Input: dimensioned drawing with shaded views. Units: mm. Origin: part minimum x, y, z. A direction names the side the tool comes from. Give positions to 0.01 mm unless a question says otherwise; leave off trailing zeros. Write each loop counter-clockwise with the first axis right and the second up, starting at its lowest first coordinate (ties: lowest second). Pieces come first, ordered by that corner, then holes. Notation, with made-up numbers: (-13.5, 88.5) - (-6.5, 88.5) arc R19 ccw to (-6.5, 99.5) - close; hole circle Ø1 at (36.25, -10.5). An arc over 180 degrees is marked (long way). Answer as CSV lines item,"result".
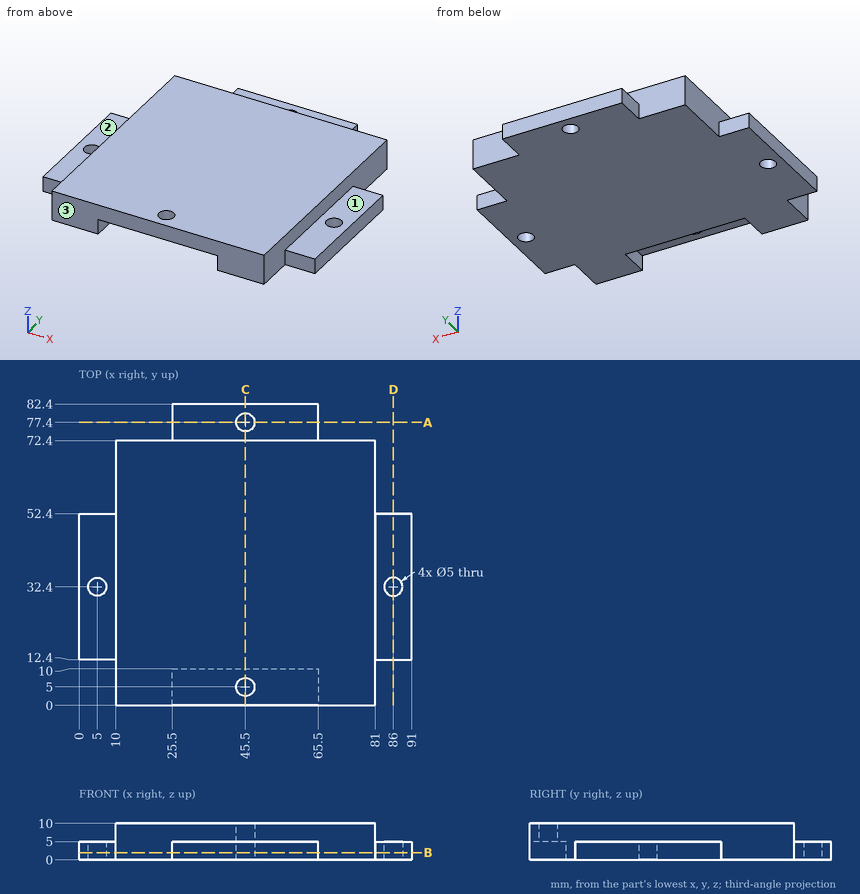
Item 1: Cut plane C-C on x = 45.5. Return the cut outline in (y, z), plus the area to 3 significant figures.
The answers:
outline,"(0, 5) - (2.5, 5) - (2.5, 10) - (0, 10) - close; (7.5, 5) - (10, 5) - (10, 0) - (74.9, 0) - (74.9, 5) - (72.4, 5) - (72.4, 10) - (7.5, 10) - close; (79.9, 0) - (82.4, 0) - (82.4, 5) - (79.9, 5) - close"
area,"674 mm²"
Item 2: Reachability of the marked faces 1, 2 and 3 from +Z, -Z, +X, -X, +Y, -Y: full face, straight path, thin tool, end or side. Return the list, or none.
The answers:
face 1,"+Z, +X, +Y, -Y"
face 2,"+Z, -X, +Y, -Y"
face 3,"+Z, -Z, +X, -X, -Y"
Item 3: Cut plane A-A on y = 77.4. Return the cut outline in (x, z).
The answers:
outline,"(25.5, 0) - (43, 0) - (43, 5) - (25.5, 5) - close; (48, 0) - (65.5, 0) - (65.5, 5) - (48, 5) - close"
Item 4: Cut plane D-D on x = 86. Return the cut outline in (y, z), plus the area to 3 significant figures.
The answers:
outline,"(12.4, 0) - (29.9, 0) - (29.9, 5) - (12.4, 5) - close; (34.9, 0) - (52.4, 0) - (52.4, 5) - (34.9, 5) - close"
area,"175 mm²"
Item 5: Cut plane B-B on z = 2. Return the cut outline in (x, y).
The answers:
outline,"(0, 12.4) - (10, 12.4) - (10, 0) - (25.5, 0) - (25.5, 10) - (65.5, 10) - (65.5, 0) - (81, 0) - (81, 12.4) - (91, 12.4) - (91, 52.4) - (81, 52.4) - (81, 72.4) - (65.5, 72.4) - (65.5, 82.4) - (25.5, 82.4) - (25.5, 72.4) - (10, 72.4) - (10, 52.4) - (0, 52.4) - close; hole circle Ø5 at (5, 32.4); hole circle Ø5 at (45.5, 77.4); hole circle Ø5 at (86, 32.4)"
Item 6: Ray query, line 1 (Y direction, x = 45.5, z = 2.2); line 2 (Y direction, x = 59, z = 1.25); line 3 (Y direction, x = 40.5, z = 9). Return the intervals inside material, ascending. Write a range as from..to.
The answers:
line 1,"10..74.9, 79.9..82.4"
line 2,"10..82.4"
line 3,"0..72.4"
Item 7: Contact query for flat-ended pins moving along their axis: pin 1 (5.5 mm diameter, centred on x = 42.5, z = 2.5, fed in from -Y); pin 2 (5.5 mm diameter, centred on x = 7.5, z = 3.5, fed in from +Y); pin 3 (6.5 mm diameter, centred on x = 45.5, y = 5, fed in from -Z); pin 4 (5.5 mm diameter, centred on y = 75.5, z = 2.5, fed in from +X). Output: stop coordinate, or through.
The answers:
pin 1,"y = 0"
pin 2,"y = 72.4"
pin 3,"z = 5"
pin 4,"x = 65.5"
